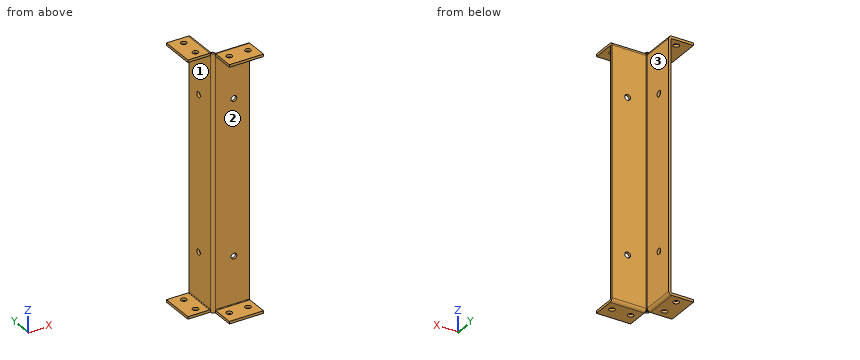
```python
from build123d import *

# Parameters (mm, degrees)
SKETCH1_W                      = 60
SKETCH1_H                      = 408
BASE_FLANGE1_DEPTH             = 4
EDGE_FLANGE1_STRIP_W           = 18
EDGE_FLANGE1_STRIP_H           = 4
EDGE_FLANGE1_STRIP_CUT_DEPTH   = 408
EDGE_FLANGE1_DEPTH             = 408
EDGE_FLANGE2_STRIP_W           = 18
EDGE_FLANGE2_STRIP_H           = 4
EDGE_FLANGE2_STRIP_CUT_DEPTH   = 55
EDGE_FLANGE2_STRIP_2_W         = 18
EDGE_FLANGE2_STRIP_2_H         = 4
EDGE_FLANGE2_STRIP_CUT_2_DEPTH = 55
EDGE_FLANGE2_STRIP_3_W         = 18
EDGE_FLANGE2_STRIP_3_H         = 4
EDGE_FLANGE2_STRIP_CUT_3_DEPTH = 55
EDGE_FLANGE2_STRIP_4_W         = 18
EDGE_FLANGE2_STRIP_4_H         = 4
EDGE_FLANGE2_STRIP_CUT_4_DEPTH = 55
EDGE_FLANGE2_DEPTH             = 55
EDGE_FLANGE2_BEND_DEPTH        = 55
EDGE_FLANGE2_BEND_2_DEPTH      = 55
EDGE_FLANGE2_BEND_3_DEPTH      = 55
SKETCH18_R                     = 4.6
EXTRUDE1_DEPTH                 = 418.636205327
SKETCH19_R                     = 4.6
EXTRUDE2_DEPTH                 = 4
SKETCH20_R                     = 4.6
EXTRUDE3_DEPTH                 = 4


# Sheet-metal steps are written as plain solids
with BuildPart() as part:
    # Sketch1 → Base-Flange1 (new body)
    with BuildSketch(Plane(origin=(0, 0, 0), x_dir=(1, 0, 0), z_dir=(0, 1, 0))):
        Rectangle(SKETCH1_W, SKETCH1_H)
    extrude(amount=BASE_FLANGE1_DEPTH)

    # Edge-Flange1 strip (across the edge) → Edge-Flange1 strip cut (cut)
    with BuildSketch(Plane(origin=(-30, 4, -204), x_dir=(1, 0, 0), z_dir=(0, 0, 1))):
        with Locations((-4, -2)):
            Rectangle(EDGE_FLANGE1_STRIP_W, EDGE_FLANGE1_STRIP_H)
    extrude(amount=EDGE_FLANGE1_STRIP_CUT_DEPTH, mode=Mode.SUBTRACT)

    # Edge-Flange1 section (across the edge) → Edge-Flange1 (add)
    with BuildSketch(Plane(origin=(-30, 4, -204), x_dir=(1, 0, 0), z_dir=(0, 0, 1))):
        with BuildLine():
            Line((0, 1), (0, 56))
            Line((0, 56), (4, 56))
            Line((4, 56), (4, 1))
            ThreePointArc((4, 1), (4.292893219, 0.292893219), (5, 0))
            Line((5, 0), (5, -4))
            ThreePointArc((5, -4), (1.464466094, -2.535533906), (0, 1))
        make_face()
    extrude(amount=EDGE_FLANGE1_DEPTH)

    # Edge-Flange2 strip (across the edge) → Edge-Flange2 strip cut (cut)
    with BuildSketch(Plane(origin=(-30, 5, 204), x_dir=(0, 0, -1), z_dir=(0, 1, 0))):
        with Locations((-4, -2)):
            Rectangle(EDGE_FLANGE2_STRIP_W, EDGE_FLANGE2_STRIP_H)
    extrude(amount=EDGE_FLANGE2_STRIP_CUT_DEPTH, mode=Mode.SUBTRACT)

    # Edge-Flange2 strip 2 (across the edge) → Edge-Flange2 strip cut 2 (cut)
    with BuildSketch(Plane(origin=(30, 0, 204), x_dir=(0, 0, -1), z_dir=(-1, 0, 0))):
        with Locations((-4, -2)):
            Rectangle(EDGE_FLANGE2_STRIP_2_W, EDGE_FLANGE2_STRIP_2_H)
    extrude(amount=EDGE_FLANGE2_STRIP_CUT_2_DEPTH, mode=Mode.SUBTRACT)

    # Edge-Flange2 strip 3 (across the edge) → Edge-Flange2 strip cut 3 (cut)
    with BuildSketch(Plane(origin=(-30, 60, -204), x_dir=(0, 0, 1), z_dir=(0, -1, 0))):
        with Locations((-4, -2)):
            Rectangle(EDGE_FLANGE2_STRIP_3_W, EDGE_FLANGE2_STRIP_3_H)
    extrude(amount=EDGE_FLANGE2_STRIP_CUT_3_DEPTH, mode=Mode.SUBTRACT)

    # Edge-Flange2 strip 4 (across the edge) → Edge-Flange2 strip cut 4 (cut)
    with BuildSketch(Plane(origin=(-25, 0, -204), x_dir=(0, 0, 1), z_dir=(1, 0, 0))):
        with Locations((-4, -2)):
            Rectangle(EDGE_FLANGE2_STRIP_4_W, EDGE_FLANGE2_STRIP_4_H)
    extrude(amount=EDGE_FLANGE2_STRIP_CUT_4_DEPTH, mode=Mode.SUBTRACT)

    # Edge-Flange2 section (across the edge) → Edge-Flange2 (add)
    with BuildSketch(Plane(origin=(-30, 5, 204), x_dir=(0, 0, -1), z_dir=(0, 1, 0))):
        with BuildLine():
            Line((0, 1), (0, 36))
            Line((0, 36), (4, 36))
            Line((4, 36), (4, 1))
            ThreePointArc((4, 1), (4.292893219, 0.292893219), (5, 0))
            Line((5, 0), (5, -4))
            ThreePointArc((5, -4), (1.464466094, -2.535533906), (0, 1))
        make_face()
    extrude(amount=EDGE_FLANGE2_DEPTH)

    # Edge-Flange2 section 2 (across the edge) → Edge-Flange2 bend (add)
    with BuildSketch(Plane(origin=(30, 0, 204), x_dir=(0, 0, -1), z_dir=(-1, 0, 0))):
        with BuildLine():
            Line((0, 1), (0, 36))
            Line((0, 36), (4, 36))
            Line((4, 36), (4, 1))
            ThreePointArc((4, 1), (4.292893219, 0.292893219), (5, 0))
            Line((5, 0), (5, -4))
            ThreePointArc((5, -4), (1.464466094, -2.535533906), (0, 1))
        make_face()
    extrude(amount=EDGE_FLANGE2_BEND_DEPTH)

    # Edge-Flange2 section 3 (across the edge) → Edge-Flange2 bend 2 (add)
    with BuildSketch(Plane(origin=(-30, 60, -204), x_dir=(0, 0, 1), z_dir=(0, -1, 0))):
        with BuildLine():
            Line((0, 1), (0, 36))
            Line((0, 36), (4, 36))
            Line((4, 36), (4, 1))
            ThreePointArc((4, 1), (4.292893219, 0.292893219), (5, 0))
            Line((5, 0), (5, -4))
            ThreePointArc((5, -4), (1.464466094, -2.535533906), (0, 1))
        make_face()
    extrude(amount=EDGE_FLANGE2_BEND_2_DEPTH)

    # Edge-Flange2 section 4 (across the edge) → Edge-Flange2 bend 3 (add)
    with BuildSketch(Plane(origin=(-25, 0, -204), x_dir=(0, 0, 1), z_dir=(1, 0, 0))):
        with BuildLine():
            Line((0, 1), (0, 36))
            Line((0, 36), (4, 36))
            Line((4, 36), (4, 1))
            ThreePointArc((4, 1), (4.292893219, 0.292893219), (5, 0))
            Line((5, 0), (5, -4))
            ThreePointArc((5, -4), (1.464466094, -2.535533906), (0, 1))
        make_face()
    extrude(amount=EDGE_FLANGE2_BEND_3_DEPTH)

    # Sketch18 → Extrude1 (cut, through all)
    with BuildSketch(Plane.XY.offset(204)):
        with Locations((-46, 47.5)):
            Circle(SKETCH18_R)
        with Locations((-46, 17.5)):
            Circle(SKETCH18_R)
        with Locations((-12.5, -16)):
            Circle(SKETCH18_R)
        with Locations((17.5, -16)):
            Circle(SKETCH18_R)
    extrude(amount=-EXTRUDE1_DEPTH, mode=Mode.SUBTRACT)

    # Sketch19 → Extrude2 (cut)
    with BuildSketch(Plane(origin=(-26, 0, 0), x_dir=(0, 0, -1), z_dir=(1, 0, 0))):
        with Locations(Location((-124, 35, 0), (0, 0, 90))):
            Circle(SKETCH19_R)
        with Locations(Location((124, 35, 0), (0, 0, 90))):
            Circle(SKETCH19_R)
    extrude(amount=-EXTRUDE2_DEPTH, mode=Mode.SUBTRACT)

    # Sketch20 → Extrude3 (cut)
    with BuildSketch(Plane(origin=(0, 4, 0), x_dir=(1, 0, 0), z_dir=(0, 1, 0))):
        with Locations(Location((5, 124, 0), (0, 0, 270))):
            Circle(SKETCH20_R)
        with Locations(Location((5, -124, 0), (0, 0, 270))):
            Circle(SKETCH20_R)
    extrude(amount=-EXTRUDE3_DEPTH, mode=Mode.SUBTRACT)


solid = part.part
```
Work out the finished part from the listing and answer in its coordinate system (mm). Face numbers are marked on the shaded views. Give positions to 0.01 mm unless a question says otherwise; leave off trailing zeros. Order: outer loops, then holes, each group sorted by start corner. A loop starts at its lowest first (then second) coordinate and runs counter-clockwise, first axis right, second up.
1. Section A-A, the plane x = 5 is taken. Determine the outline of the cut face in (y, z).
Result sheet:
outline: (-36, -204) - (-1, -204) arc R5 ccw to (4, -199) - (4, -128.6) - (0, -128.6) - (0, -199) arc R1 cw to (-1, -200) - (-36, -200) - close; (-36, 200) - (-1, 200) arc R1 cw to (0, 199) - (0, 128.6) - (4, 128.6) - (4, 199) arc R5 ccw to (-1, 204) - (-36, 204) - close; (0, -119.4) - (4, -119.4) - (4, 119.4) - (0, 119.4) - close
2. The mould has two halves that part along Z. Classify the marked faces 1, 2 and 3: released by +Z, released by -Z, zero draft, split by the parting line, or undercut.
Result sheet:
face 1: undercut
face 2: undercut
face 3: zero draft
3. Section B-B, the plane y = 47.5 is taken. Determine the outline of the cut face in (x, z), and give its area (3 significant figures).
Result sheet:
outline: (-66, -204) - (-50.6, -204) - (-50.6, -200) - (-66, -200) - close; (-66, 200) - (-50.6, 200) - (-50.6, 204) - (-66, 204) - close; (-41.4, -204) - (-31, -204) arc R5 ccw to (-26, -199) - (-26, 199) arc R5 ccw to (-31, 204) - (-41.4, 204) - (-41.4, 200) - (-31, 200) arc R1 cw to (-30, 199) - (-30, -199) arc R1 cw to (-31, -200) - (-41.4, -200) - close
area: 1,840 mm2
4. Straight lines are drawn through the part: L1, parallel to Y at x = -46, z = 201.25; L2, parallel to Z at x = -41.5, y = 56.5; L3, parallel to Y at x = 2.5, z = 106.5. For each, find the intervals that lie inside material, in ascending order.
Result sheet:
L1: y = 5 to 12.9, 22.1 to 42.9, 52.1 to 60
L2: z = -204 to -200, 200 to 204
L3: y = 0 to 4
5. Section C-C, the plane z = -124 is taken. Determine the outline of the cut face in (x, y), and give its area (3 significant figures).
Result sheet:
outline: (-30, 5) arc R5 ccw to (-25, 0) - (0.4, 0) - (0.4, 4) - (-25, 4) arc R1 cw to (-26, 5) - (-26, 30.4) - (-30, 30.4) - close; (-30, 39.6) - (-26, 39.6) - (-26, 60) - (-30, 60) - close; (9.6, 0) - (30, 0) - (30, 4) - (9.6, 4) - close
area: 385 mm2
6. Section D-D, the plane x = -46 is taken. Determine the outline of the cut face in (y, z).
Result sheet:
outline: (5, -204) - (12.9, -204) - (12.9, -200) - (5, -200) - close; (5, 200) - (12.9, 200) - (12.9, 204) - (5, 204) - close; (22.1, -204) - (42.9, -204) - (42.9, -200) - (22.1, -200) - close; (22.1, 200) - (42.9, 200) - (42.9, 204) - (22.1, 204) - close; (52.1, -204) - (60, -204) - (60, -200) - (52.1, -200) - close; (52.1, 200) - (60, 200) - (60, 204) - (52.1, 204) - close
7. Each of these flat-tipped pins is pushed along its axis until it touches: P1, Ø2, axis at x = -8, z = -85, coming from the -Y side; P2, Ø2, axis at y = 50, z = -126.5, coming from the -X side; P3, Ø4, axis at x = -27.5, y = -2, coming from the +Z side; P4, Ø5.5, axis at y = -10.5, z = 200.5, coming from the -X side. Where does it stop, or does it pass through?
Result sheet:
P1: stops at y = 0
P2: stops at x = -30
P3: passes through
P4: stops at x = -25
